```python
from build123d import *

# Parameters (mm, degrees)
SKETCH1_W           = 60
SKETCH1_H           = 28
SKETCH1_W_2         = 40
SKETCH1_H_2         = 20
BOSS_EXTRUDE1_DEPTH = 32
SKETCH2_W           = 60
SKETCH2_H           = 28
BOSS_EXTRUDE2_DEPTH = 4
SKETCH3_W           = 30
SKETCH3_H           = 28
SKETCH3_R           = 5.5
BOSS_EXTRUDE3_DEPTH = 4
SKETCH4_R           = 1.95
CUT_EXTRUDE1_DEPTH  = 4
SKETCH5_R           = 2.2
CUT_EXTRUDE2_DEPTH  = 15


with BuildPart() as part:
    # Sketch1 → Boss-Extrude1 (new body)
    with BuildSketch(Plane.XY):
        with Locations((20, -10)):
            Rectangle(SKETCH1_W, SKETCH1_H)
        with Locations((20, -10)):
            Rectangle(SKETCH1_W_2, SKETCH1_H_2, mode=Mode.SUBTRACT)
    extrude(amount=BOSS_EXTRUDE1_DEPTH)

    # Sketch2 → Boss-Extrude2 (add)
    with BuildSketch(Plane.XY.offset(32)):
        with Locations((20, -10)):
            Rectangle(SKETCH2_W, SKETCH2_H)
    extrude(amount=BOSS_EXTRUDE2_DEPTH)

    # Sketch3 → Boss-Extrude3 (add)
    with BuildSketch(Plane(origin=(50, 0, 0), x_dir=(0, 0, -1), z_dir=(1, 0, 0))):
        with Locations((-51, -10)):
            Rectangle(SKETCH3_W, SKETCH3_H)
        with Locations((-51, -10)):
            Circle(SKETCH3_R, mode=Mode.SUBTRACT)
    extrude(amount=-BOSS_EXTRUDE3_DEPTH)

    # Sketch4 → Cut-Extrude1 (cut)
    with BuildSketch(Plane(origin=(50, 0, 0), x_dir=(0, 0, -1), z_dir=(1, 0, 0))):
        with Locations((-51, -18)):
            Circle(SKETCH4_R)
        with Locations((-59, -10)):
            Circle(SKETCH4_R)
        with Locations((-43, -10)):
            Circle(SKETCH4_R)
        with Locations((-51, -2)):
            Circle(SKETCH4_R)
    extrude(amount=-CUT_EXTRUDE1_DEPTH, mode=Mode.SUBTRACT)

    # Sketch5 → Cut-Extrude2 (cut)
    with BuildSketch(Plane(origin=(0, 0, 0), x_dir=(-1, 0, 0), z_dir=(0, 0, -1))):
        with Locations((-44.4, -5)):
            Circle(SKETCH5_R)
        with Locations((-44.4, -15)):
            Circle(SKETCH5_R)
        with Locations((4.4, -5)):
            Circle(SKETCH5_R)
        with Locations((4.4, -15)):
            Circle(SKETCH5_R)
    extrude(amount=-CUT_EXTRUDE2_DEPTH, mode=Mode.SUBTRACT)


solid = part.part
```
The model under review builds one solid part; all positions refer to its coordinate system, in mm. A direction names the side the tool comes from. Coordinates: 2 decimals unless noted, no trailing zeros. Order: outer loops, then holes, each group sorted by start corner. A loop starts at its lowest first (then second) coordinate and runs counter-clockwise, first axis right, second up. Notation, with made-up numbers: (26.5, 28.25) -> (65.5, 28.25) arc R18 ccw to (65.5, 40.25) -> close; hole circle Ø4 at (-9, 24.25). An arc over 180 degrees is marked (long way). Answer in a Markdown table with one row per item. Add a question column.
Item 1: Mouldability with a two-part tool opening along Z and no side actions: class faces 1 (the flat face through (44, -15, 15)), 2 (the cylindrical face through (48.03, -10.75, 57.2)), 3 (the flat face through (46, -16, 55)) as +Z half, -Z half, draft (parallel to the pull), parting line (faces both ways), or undercut.
Item 2: We need section C-C on x = 44.4. Write out the cut boundary in (y, z).
Item 3: We need section A-A on z = 43. Write out the cut boundary in (x, y), plus the area to 3 significant figures.
Item 4: Machinability: for faces 4 (the flat face through (18, -10, 36)), 5 (the flat face through (0, -10, 16)), 6 (the cylindrical face through (48.03, -18.75, 49.2)), which of the approach directions +Z, -Z, +X, -X, +Y, -Y give a long, thin tool a straight path to every point of the face, cutting with its end or side? Answer none if there is none.
Item 5: We need section B-B on y = -2. Write out the cut boundary in (x, z).
Item 6: Clearance check with flat-ended pins moving along their axes: pin 1 (5 mm diameter, centred on x = -4.4, y = -15, fed in from -Z); pin 2 (1.5 mm diameter, centred on x = 25.5, y = -18.5, fed in from -Z); pin 3 (5.5 mm diameter, centred on x = -4.4, y = -5, fed in from +Z); pin 4 (1.3 mm diameter, centred on x = 45.5, y = -15, fed in from -Z). State where each tip first meets the part, or that it passes through.
Item 7: To check wall thickness, follow probe 1 along Y at (x, z) = (44.4, 7.75); probe 2 along X at (y, z) = (-5.75, 6); probe 3 along X at (y, z) = (-1.25, 22). State the ranges of each line that lie inside material, in increasing order.
Item 8: We need section D-D on y = -10. Write out the cut boundary in (x, z), plus the area to 3 significant figures.
Final values:
| question | item | result |
|---|---|---|
| 1 | face 1 | -Z half |
| 1 | face 2 | undercut |
| 1 | face 3 | draft |
| 2 | outline | (-24, 0) -> (-17.2, 0) -> (-17.2, 15) -> (-12.8, 15) -> (-12.8, 0) -> (-7.2, 0) -> (-7.2, 15) -> (-2.8, 15) -> (-2.8, 0) -> (4, 0) -> (4, 36) -> (-24, 36) -> close |
| 3 | outline | (46, -24) -> (50, -24) -> (50, -11.95) -> (46, -11.95) -> close; (46, -8.05) -> (50, -8.05) -> (50, 4) -> (46, 4) -> close |
| 3 | area | 96.4 mm2 |
| 4 | face 4 | +Z, -X, +Y, -Y |
| 4 | face 5 | -Z |
| 4 | face 6 | +X, -X |
| 5 | outline | (-10, 0) -> (0, 0) -> (0, 32) -> (40, 32) -> (40, 0) -> (50, 0) -> (50, 49.05) -> (46, 49.05) -> (46, 36) -> (-10, 36) -> close; (46, 52.95) -> (50, 52.95) -> (50, 66) -> (46, 66) -> close |
| 6 | pin 1 | stops at z = 0 |
| 6 | pin 2 | stops at z = 32 |
| 6 | pin 3 | stops at z = 36 |
| 6 | pin 4 | stops at z = 15 |
| 7 | probe 1 | y = -24 to -17.2, -12.8 to -7.2, -2.8 to 4 |
| 7 | probe 2 | x = -10 to -6.47, -2.33 to 0, 40 to 42.33, 46.47 to 50 |
| 7 | probe 3 | x = -10 to 0, 40 to 50 |
| 8 | outline | (-10, 0) -> (0, 0) -> (0, 32) -> (40, 32) -> (40, 0) -> (50, 0) -> (50, 41.05) -> (46, 41.05) -> (46, 36) -> (-10, 36) -> close; (46, 44.95) -> (50, 44.95) -> (50, 45.5) -> (46, 45.5) -> close; (46, 56.5) -> (50, 56.5) -> (50, 57.05) -> (46, 57.05) -> close; (46, 60.95) -> (50, 60.95) -> (50, 66) -> (46, 66) -> close |
| 8 | area | 925 mm2 |
